For this review, use the dimensioned drawing (mm, ordinates from the lowest corner) and the shaded views. Give positions to 0.01 mm unless a question says otherwise; leave off trailing zeros. Write each loop counter-clockwise with the first axis right and the second up, starting at its lowest first coordinate (ties: lowest second). Pieces come first, ordered by that corner, then holes. Notation, with made-up numbers: M 19,3.5 L 38,3.5 A30 ccw 38,40.5 Z; hole C 60.5,-39.75 d9. An arc over 180 degrees is marked long. One line per item, written item: value. Start each with the question number.
Item 1: Consider section A-A, the plane x = 15.5. Write out the cut boundary in (y, z).
Item 2: Clearance check with flat-ended pins moving along their axes: pin 1 Ø17 at (x, y) = (15.5, 15.5) entering from -Z; pin 2 Ø5 at (x, z) = (7.5, 5) entering from -Y; pin 3 Ø2 at (x, y) = (27, 8.5) entering from -Z; pin 4 Ø4 at (y, z) = (4.5, 1) entering from +X. State where each tip first meets the part, or that it passes through.
Item 3: Consider section D-D, the plane y = 26. Write out the cut boundary in (x, z).
Item 4: Mouldability with a two-part tool opening along Y and no side actions: class the marked faces 1, 2 and 3 as released by +Y, released by -Y, zero draft, split by the parting line, or undercut.
Item 5: Consider section C-C, the plane z = 4.25. Write out the cut boundary in (x, y), and give its area (3 significant figures).
Item 6: To check wall thickness, follow probe 1 along Y at (x, z) = (15.5, 0.35); probe 2 along Y at (x, z) = (15.5, 5.5); probe 3 along Z at (x, y) = (12, 2). State the ranges of each line that lie inside material, in increasing order.
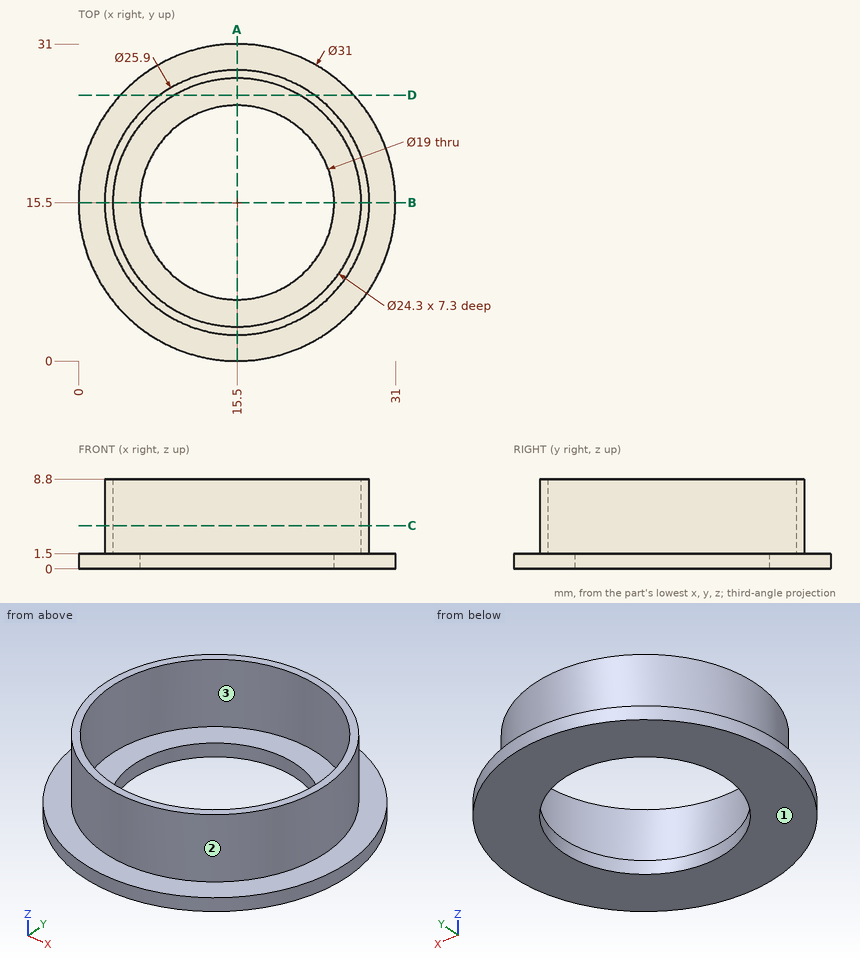
Model answer:
1. outline: M 0,0 L 6,0 L 6,1.5 L 3.35,1.5 L 3.35,8.8 L 2.55,8.8 L 2.55,1.5 L 0,1.5 Z; M 25,0 L 31,0 L 31,1.5 L 28.45,1.5 L 28.45,8.8 L 27.65,8.8 L 27.65,1.5 L 25,1.5 Z
2. pin 1: passes through
2. pin 2: stops at y = 3.78
2. pin 3: stops at z = 0
2. pin 4: stops at x = 28.12
3. outline: M 4.1,0 L 26.9,0 L 26.9,1.5 L 23.08,1.5 L 23.08,8.8 L 21.61,8.8 L 21.61,1.5 L 9.39,1.5 L 9.39,8.8 L 7.92,8.8 L 7.92,1.5 L 4.1,1.5 Z
4. face 1: zero draft
4. face 2: split by the parting line
4. face 3: undercut
5. outline: C 15.5,15.5 d25.9; hole C 15.5,15.5 d24.3
5. area: 63.1 mm2
6. probe 1: y = 0 to 6, 25 to 31
6. probe 2: y = 2.55 to 3.35, 27.65 to 28.45
6. probe 3: z = 0 to 1.5
